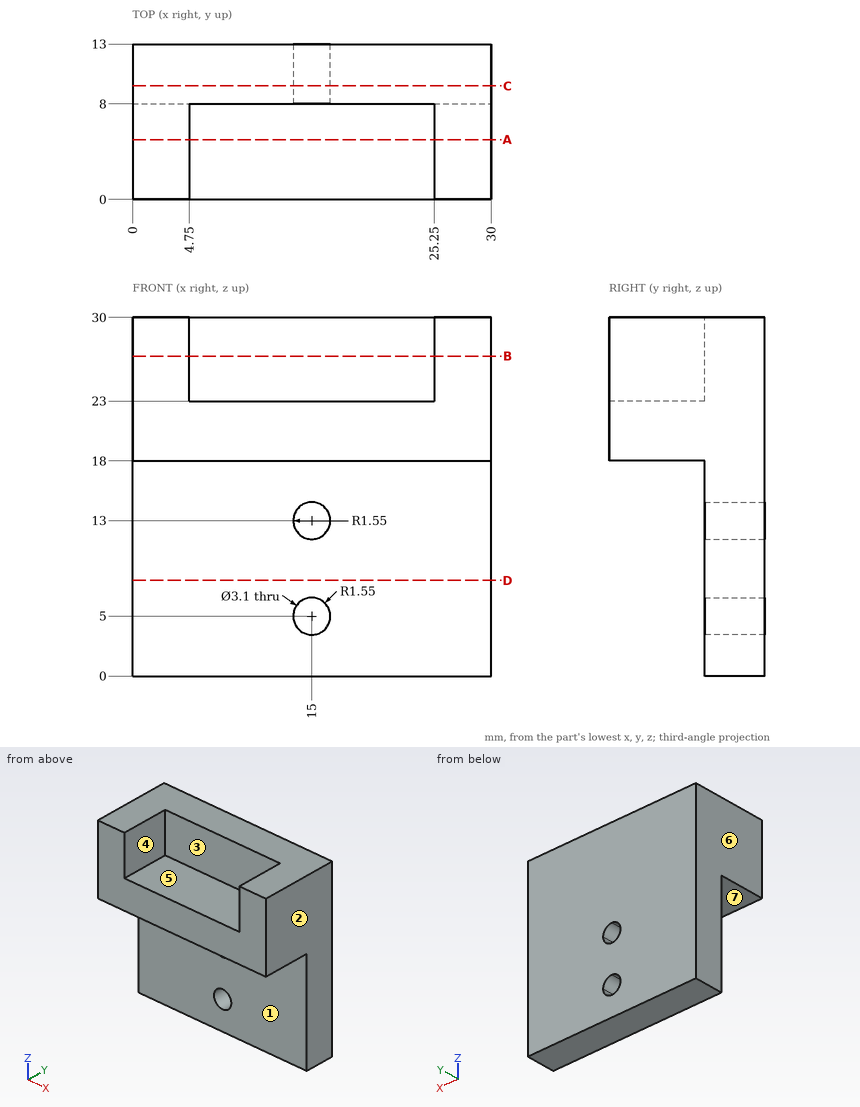
Answer from the drawing. Dimensions are ordinates in mm from the lowest x, y and z of the part. A direction names the side the tool comes from. Round coordinates to 2 decimals unless told otherwise and drop trailing zeros. Write each loop counter-clockwise with the first axis right and the second up, starting at its lowest first coordinate (ties: lowest second). Pieces come first, ordered by that corner, then holes.
1. Straight lines are drawn through the part: L1, parallel to Z at x = 15, y = 11.55; L2, parallel to X at y = 10.75, z = 5; L3, parallel to Y at x = 6.5, z = 2.25. For each, find the intervals that lie inside material, in ascending order.
2. The part is cut by section C-C, the plane y = 9.5. Determine the outline of the cut face in (x, z), then the cut area to 3 significant figures.
3. Determine the mould class of the marked faces 4, 5, 6 and 7 for opening direction X: pulls with the +X half, pulls with the -X half, needs draft (parallel to the pull), parting line crosses it, or undercut.
4. The part is cut by section B-B, the plane z = 26.75. Determine the outline of the cut face in (x, y), then the cut area to 3 significant figures.
5. Given pin 1 Ø7.5 at (y, z) = (5.5, 25) entering from -X; pin 2 Ø4 at (x, y) = (19.5, 1.5) entering from +Z; pin 3 Ø5.5 at (x, z) = (11, 26.5) entering from -Y; pin 4 Ø4 at (x, y) = (11, 5) entering from -Z, each flat-ended and moving along its own axis, determine where each tip first touches the part or whether it passes through.
6. Which of the six approach directions +Z, -Z, +X, -X, +Y, -Y give full straight-line access (tool end or side, diameter ignored) to the marked faces 1, 2 and 3?
7. The part is cut by section A-A, the plane y = 5. Determine the outline of the cut face in (x, z), then the cut area to 4 significant figures.
8. The part is cut by section D-D, the plane z = 8. Determine the outline of the cut face in (x, y), then the cut area to 3 significant figures.
Values:
1. L1: z = 0 to 3.45, 6.55 to 11.45, 14.55 to 30
1. L2: x = 0 to 13.45, 16.55 to 30
1. L3: y = 8 to 13
2. outline: (0, 0) - (30, 0) - (30, 30) - (0, 30) - close; hole circle Ø3.1 at (15, 5); hole circle Ø3.1 at (15, 13)
2. area: 885 mm2
3. face 4: undercut
3. face 5: undercut
3. face 6: pulls with the -X half
3. face 7: needs draft
4. outline: (0, 0) - (4.75, 0) - (4.75, 8) - (25.25, 8) - (25.25, 0) - (30, 0) - (30, 13) - (0, 13) - close
4. area: 226 mm2
5. pin 1: stops at x = 0
5. pin 2: stops at z = 23
5. pin 3: stops at y = 8
5. pin 4: stops at z = 18
6. face 1: -Z, +X, -X, -Y
6. face 2: +Z, -Z, +X, +Y, -Y
6. face 3: +Z, -Y
7. outline: (0, 18) - (30, 18) - (30, 30) - (25.25, 30) - (25.25, 23) - (4.75, 23) - (4.75, 30) - (0, 30) - close
7. area: 216.5 mm2
8. outline: (0, 8) - (30, 8) - (30, 13) - (0, 13) - close
8. area: 150 mm2
